from build123d import *

# Parameters (mm, degrees)
F1_DEPTH = 177.8
F2_R     = 6.35
F3_DEPTH = 25.4
F4_W     = 165.1
F4_H     = 19.05
F5_DEPTH = 76.201
F6_R     = 6.35
F7_DEPTH = 25.4


with BuildPart() as f1:
    # F0 (on Right) → F1 (new body, symmetric)
    with BuildSketch(Plane.YZ):
        with BuildLine():
            Line((0, 0), (0, 76.2))
            ThreePointArc((0, 76.2), (-6.7351920908, 73.4101920908), (-9.525, 66.675))
            Line((-9.525, 66.675), (-9.525, 19.05))
            ThreePointArc((-9.525, 19.05), (-12.3148079092, 12.3148079092), (-19.05, 9.525))
            Line((-19.05, 9.525), (-79.375, 9.525))
            ThreePointArc((-79.375, 9.525), (-86.1101920908, 6.7351920908), (-88.9, 0))
            Line((-88.9, 0), (0, 0))
        make_face()
    extrude(amount=F1_DEPTH, both=True)

    # F2 (on face) → F3 (cut)
    with BuildSketch(Plane(origin=(0, 0, 0), x_dir=(-1, 0, 0), z_dir=(0, 1, 0))):
        with Locations((127, 38.1)):
            Circle(F2_R)
        with Locations((50.8, 38.1)):
            Circle(F2_R)
    extrude(amount=-F3_DEPTH, mode=Mode.SUBTRACT)

    # F4 (on face) → F5 (cut, through all)
    with BuildSketch(Plane(origin=(0, 0, 0), x_dir=(1, 0, 0), z_dir=(0, 0, -1))):
        with Locations((95.25, 9.525)):
            Rectangle(F4_W, F4_H)
    extrude(amount=-F5_DEPTH, mode=Mode.SUBTRACT)

    # F6 (on face) → F7 (cut)
    with BuildSketch(Plane(origin=(0, 0, 0), x_dir=(1, 0, 0), z_dir=(0, 0, -1))):
        with Locations((127, 49.2125)):
            Circle(F6_R)
    extrude(amount=-F7_DEPTH, mode=Mode.SUBTRACT)


solid = f1.part
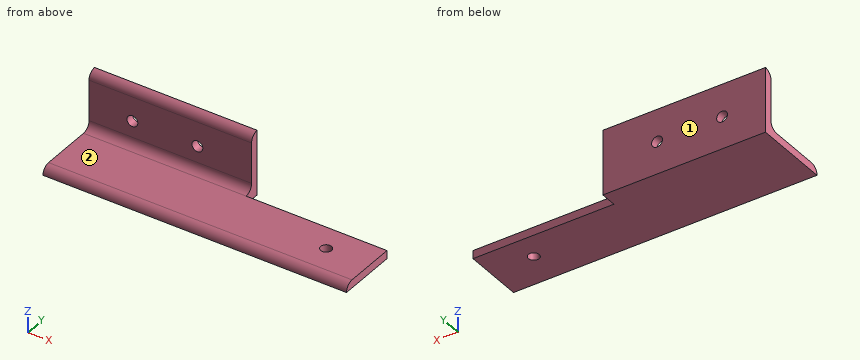
Part model, mm, in its own coordinate system. Face numbers are marked on the shaded views. A direction names the side the tool comes from. Give positions to 0.01 mm unless a question says otherwise; leave off trailing zeros. Write each loop counter-clockwise with the first axis right and the second up, starting at its lowest first coordinate (ties: lowest second). Pieces come first, ordered by that corner, then holes.
1) Which spindle directions (+Z, -Z, +X, -X, +Y, -Y) get a long thin tool onto all of the face, cutting with end or side? Do the marked faces 1 and 2. Say none if no direction does.
Resolved:
face 1: +Z, -Z, +X, -X, +Y
face 2: +Z, +X, -X, -Y
2) Probe L1, parallel to X at y = -6, z = 38; L2, parallel to Z at x = 69, y = -75 (3 decimals); L3, parallel to Z at x = -50.8, y = -3.25. List the from-to ranges inside material, lowest first.
Resolved:
L1: x = -177.8 to -133.35, -120.65 to -57.15, -44.45 to 12.7
L2: z = 0 to 9.525
L3: z = 0 to 31.75, 44.45 to 75.63
3) Cut at D-D on y = -38. Write the cut outline in (x, z) (3 decimals), then the cut area to 3 significant figures.
Resolved:
outline: (-177.8, 0) - (177.8, 0) - (177.8, 9.525) - (-177.8, 9.525) - close
area: 3,390 mm2
4) Cut at C-C on x = -13. Write the cut outline in (y, z) (3 decimals).
Resolved:
outline: (-88.9, 0) - (0, 0) - (0, 76.2) arc R9.525 ccw to (-9.525, 66.675) - (-9.525, 19.05) arc R9.525 cw to (-19.05, 9.525) - (-79.375, 9.525) arc R9.525 ccw to start
5) Pin check, flat tips, straight feed: pin 1 (10 mm diameter, centred on x = -50.8, z = 38.1, fed in from +Y); pin 2 (5 mm diameter, centred on x = -104, z = 60, fed in from -Y) (3 decimals); pin 3 (21 mm diameter, centred on y = -5.5, z = 40.5, fed in from +X); pin 4 (5 mm diameter, centred on x = -95.5, y = -13.5, fed in from +Z). Stop position of each tip, or through.
Resolved:
pin 1: passes through
pin 2: stops at y = -9.525
pin 3: stops at x = 12.7
pin 4: stops at z = 13.96
6) Cut at A-A on z = 38.1. Write the cut outline in (x, y) (3 decimals), then the cut area to 3 significant figures.
Resolved:
outline: (-177.8, -9.525) - (-133.35, -9.525) - (-133.35, 0) - (-177.8, 0) - close; (-120.65, -9.525) - (-57.15, -9.525) - (-57.15, 0) - (-120.65, 0) - close; (-44.45, -9.525) - (12.7, -9.525) - (12.7, 0) - (-44.45, 0) - close
area: 1,570 mm2
